Geometry check sheet. Reference: the model listing, model coordinates, mm. Round coordinates to 2 decimals unless told otherwise and drop trailing zeros. Order: outer loops, then holes, each group sorted by start corner. A loop starts at its lowest first (then second) coordinate and runs counter-clockwise, first axis right, second up. Notation, with made-up numbers: (-34, 13.5) - (-27, 13.5) arc R17 ccw to (-27, 32.5) - close; hole circle Ø4 at (74.25, -4.75). An arc over 180 degrees is marked (long way). One line per question, with ' | ' between items. Start each with the question number.
Q1. Sectioned sample at C-C, the plane x = -2.75. Enter the section's corners in (y, z), then the cut area to 3 significant figures.
Q2. Mould release check, pull along X, two halves, no side actions. Record for faces 1 (the face through (-2.5, 2.5, 0.1)), 2 (the face through (2, 0, 0)), 3 (the face through (1.5, 2, 0)): +X half, -X half, draft (parallel to the pull), parting line (faces both ways), or undercut.
Q3. Material ranges on line 1 along X through (y, z) = (1.75, -4); line 2 along X through (y, z) = (2.9, 1); line 3 along Z through (x, y) = (1, 1.75), recorded low to high.
Q4. Sectioned sample at D-D, the plane x = 2.5. Enter the section's corners in (y, z), then the cut area to 3 significant figures.
Q5. Gauge pin test, flat ends, axial feed: P1, Ø3, axis at x = -1, z = -1.5, coming from the +Y side; P2, Ø1.5, axis at x = -3, y = 4, coming from the +Z side. Record the tip position at first contact, or that the pin passes through.
Q6. Sectioned sample at B-B, the plane x = 0. Enter the section's corners in (y, z), then the cut area to 3 significant figures.
Q7. Sectioned sample at A-A, the plane z = 0. Enter the section's corners in (x, y) (3 decimals).
```python
from build123d import *

# Parameters (mm, degrees)
BOSS_EXTRUDE1_DEPTH = 5
CIRPATTERN1_DEPTH   = 5


# Read off the part's stored shape, not the designer's step: CirPattern1
with BuildPart() as part:
    # Sketch2 → Boss-Extrude1 (new body)
    with BuildSketch(Plane(origin=(0, 0, 0), x_dir=(1, 0, 0), z_dir=(0, 1, 0))):
        with BuildLine():
            Line((-0.3925, 3.98069639), (-0.6, 3.321238474))
            ThreePointArc((-0.6, 3.321238474), (0, -3.375), (0.6, 3.321238474))
            Line((0.6, 3.321238474), (0.3925, 3.98069639))
            Line((0.3925, 3.98069639), (0.25, 4.493050189))
            ThreePointArc((0.25, 4.493050189), (0, 4.5), (-0.25, 4.493050189))
            Line((-0.25, 4.493050189), (-0.3925, 3.98069639))
        make_face()
        with BuildLine():
            Line((1.5, 2), (1.5, -2))
            ThreePointArc((1.5, -2), (-2.5, 0), (1.5, 2))
        make_face(mode=Mode.SUBTRACT)
    extrude(amount=BOSS_EXTRUDE1_DEPTH)

    # CirPattern1 outline → CirPattern1 (add)
    with BuildSketch(Plane(origin=(0, 0, 0), x_dir=(1, 0, 0), z_dir=(0, 1, 0))):
        with BuildLine():
            Line((1.724219199, 4.156569277), (1.373529153, 3.756782888))
            Line((1.373529153, 3.756782888), (0.900450047, 3.252662711))
            ThreePointArc((0.900450047, 3.252662711), (1.46435762, 3.040769929), (1.981612688, 2.732002224))
            Line((1.981612688, 2.732002224), (2.080789715, 3.416184152))
            Line((2.080789715, 3.416184152), (2.174703633, 3.939627407))
            ThreePointArc((2.174703633, 3.939627407), (1.952476826, 4.054359906), (1.724219199, 4.156569277))
        make_face()
        with BuildLine():
            Line((-2.080789715, 3.416184152), (-1.981612688, 2.732002224))
            ThreePointArc((-1.981612688, 2.732002224), (-1.46435762, 3.040769929), (-0.900450047, 3.252662711))
            Line((-0.900450047, 3.252662711), (-1.373529153, 3.756782888))
            Line((-1.373529153, 3.756782888), (-1.724219199, 4.156569277))
            ThreePointArc((-1.724219199, 4.156569277), (-1.952476826, 4.054359906), (-2.174703633, 3.939627407))
            Line((-2.174703633, 3.939627407), (-2.080789715, 3.416184152))
        make_face()
        with BuildLine():
            Line((-3.356953507, 2.175054747), (-2.970742681, 1.601659428))
            ThreePointArc((-2.970742681, 1.601659428), (-2.638681254, 2.104278081), (-2.222554919, 2.539857207))
            Line((-2.222554919, 2.539857207), (-2.867514013, 2.78879246))
            Line((-2.867514013, 2.78879246), (-3.35693564, 2.996828843))
            ThreePointArc((-3.35693564, 2.996828843), (-3.518241671, 2.805704108), (-3.66868054, 2.605913101))
            Line((-3.66868054, 2.605913101), (-3.356953507, 2.175054747))
        make_face()
        with BuildLine():
            Line((-3.968231487, 0.503129073), (-3.371480652, 0.15408834))
            ThreePointArc((-3.371480652, 0.15408834), (-3.290381704, 0.751008152), (-3.104455531, 1.324001834))
            Line((-3.104455531, 1.324001834), (-3.793552554, 1.268447484))
            Line((-3.793552554, 1.268447484), (-4.324769807, 1.243529702))
            ThreePointArc((-4.324769807, 1.243529702), (-4.387175605, 1.001344203), (-4.436030273, 0.756065746))
            Line((-4.436030273, 0.756065746), (-3.968231487, 0.503129073))
        make_face()
        with BuildLine():
            Line((-3.793552554, -1.268447484), (-3.104455531, -1.324001834))
            ThreePointArc((-3.104455531, -1.324001834), (-3.290381704, -0.751008152), (-3.371480652, -0.15408834))
            Line((-3.371480652, -0.15408834), (-3.968231487, -0.503129073))
            Line((-3.968231487, -0.503129073), (-4.436030273, -0.756065746))
            ThreePointArc((-4.436030273, -0.756065746), (-4.387175605, -1.001344203), (-4.324769807, -1.243529702))
            Line((-4.324769807, -1.243529702), (-3.793552554, -1.268447484))
        make_face()
        with BuildLine():
            Line((-2.867514013, -2.78879246), (-2.222554919, -2.539857207))
            ThreePointArc((-2.222554919, -2.539857207), (-2.638681254, -2.104278081), (-2.970742681, -1.601659428))
            Line((-2.970742681, -1.601659428), (-3.356953507, -2.175054747))
            Line((-3.356953507, -2.175054747), (-3.66868054, -2.605913101))
            ThreePointArc((-3.66868054, -2.605913101), (-3.518241671, -2.805704108), (-3.35693564, -2.996828843))
            Line((-3.35693564, -2.996828843), (-2.867514013, -2.78879246))
        make_face()
        with BuildLine():
            Line((-1.373529153, -3.756782888), (-0.900450047, -3.252662711))
            ThreePointArc((-0.900450047, -3.252662711), (-1.46435762, -3.040769929), (-1.981612688, -2.732002224))
            Line((-1.981612688, -2.732002224), (-2.080789715, -3.416184152))
            Line((-2.080789715, -3.416184152), (-2.174703633, -3.939627407))
            ThreePointArc((-2.174703633, -3.939627407), (-1.952476826, -4.054359906), (-1.724219199, -4.156569277))
            Line((-1.724219199, -4.156569277), (-1.373529153, -3.756782888))
        make_face()
        with BuildLine():
            Line((0.3925, -3.98069639), (0.6, -3.321238474))
            ThreePointArc((0.6, -3.321238474), (0, -3.375), (-0.6, -3.321238474))
            Line((-0.6, -3.321238474), (-0.3925, -3.98069639))
            Line((-0.3925, -3.98069639), (-0.25, -4.493050189))
            ThreePointArc((-0.25, -4.493050189), (0, -4.5), (0.25, -4.493050189))
            Line((0.25, -4.493050189), (0.3925, -3.98069639))
        make_face()
        with BuildLine():
            Line((2.080789715, -3.416184152), (1.981612688, -2.732002224))
            ThreePointArc((1.981612688, -2.732002224), (1.46435762, -3.040769929), (0.900450047, -3.252662711))
            Line((0.900450047, -3.252662711), (1.373529153, -3.756782888))
            Line((1.373529153, -3.756782888), (1.724219199, -4.156569277))
            ThreePointArc((1.724219199, -4.156569277), (1.952476826, -4.054359906), (2.174703633, -3.939627407))
            Line((2.174703633, -3.939627407), (2.080789715, -3.416184152))
        make_face()
        with BuildLine():
            Line((3.356953507, -2.175054747), (2.970742681, -1.601659428))
            ThreePointArc((2.970742681, -1.601659428), (2.638681254, -2.104278081), (2.222554919, -2.539857207))
            Line((2.222554919, -2.539857207), (2.867514013, -2.78879246))
            Line((2.867514013, -2.78879246), (3.35693564, -2.996828843))
            ThreePointArc((3.35693564, -2.996828843), (3.518241671, -2.805704108), (3.66868054, -2.605913101))
            Line((3.66868054, -2.605913101), (3.356953507, -2.175054747))
        make_face()
        with BuildLine():
            Line((3.968231487, -0.503129073), (3.371480652, -0.15408834))
            ThreePointArc((3.371480652, -0.15408834), (3.290381704, -0.751008152), (3.104455531, -1.324001834))
            Line((3.104455531, -1.324001834), (3.793552554, -1.268447484))
            Line((3.793552554, -1.268447484), (4.324769807, -1.243529702))
            ThreePointArc((4.324769807, -1.243529702), (4.387175605, -1.001344203), (4.436030273, -0.756065746))
            Line((4.436030273, -0.756065746), (3.968231487, -0.503129073))
        make_face()
        with BuildLine():
            Line((3.793552554, 1.268447484), (3.104455531, 1.324001834))
            ThreePointArc((3.104455531, 1.324001834), (3.290381704, 0.751008152), (3.371480652, 0.15408834))
            Line((3.371480652, 0.15408834), (3.968231487, 0.503129073))
            Line((3.968231487, 0.503129073), (4.436030273, 0.756065746))
            ThreePointArc((4.436030273, 0.756065746), (4.387175605, 1.001344203), (4.324769807, 1.243529702))
            Line((4.324769807, 1.243529702), (3.793552554, 1.268447484))
        make_face()
        with BuildLine():
            Line((2.867514013, 2.78879246), (2.222554919, 2.539857207))
            ThreePointArc((2.222554919, 2.539857207), (2.638681254, 2.104278081), (2.970742681, 1.601659428))
            Line((2.970742681, 1.601659428), (3.356953507, 2.175054747))
            Line((3.356953507, 2.175054747), (3.66868054, 2.605913101))
            ThreePointArc((3.66868054, 2.605913101), (3.518241671, 2.805704108), (3.35693564, 2.996828843))
            Line((3.35693564, 2.996828843), (2.867514013, 2.78879246))
        make_face()
    extrude(amount=CIRPATTERN1_DEPTH)


solid = part.part
```
Determined:
1) outline: (0, -2.74) - (5, -2.74) - (5, 2.74) - (0, 2.74) - close | area: 27.4 mm2
2) face 1: undercut | face 2: draft | face 3: undercut
3) line 1: x = -2.06 to -1.59, -0.39 to 0.39, 1.59 to 2.06 | line 2: x = -4.39 to -2.29, 1.5 to 4.39 | line 3: z = -3.36 to -2.29, 2.29 to 3.36
4) outline: (0, -2.65) - (5, -2.65) - (5, 2.65) - (0, 2.65) - close | area: 26.5 mm2
5) P1: stops at y = 5 | P2: stops at z = 3
6) outline: (0, -4.5) - (5, -4.5) - (5, -2.5) - (0, -2.5) - close; (0, 2.5) - (5, 2.5) - (5, 4.5) - (0, 4.5) - close | area: 20.0 mm2
7) outline: (-3.375, 0) - (-2.5, 0) - (-2.5, 5) - (-3.375, 5) - close; (1.5, 0) - (3.375, 0) - (3.375, 5) - (1.5, 5) - close
